Verification items for this drawing (mm, ordinates from the low corner). A direction names the side the tool comes from. Round coordinates to 2 decimals unless told otherwise and drop trailing zeros. Order: outer loops, then holes, each group sorted by start corner. A loop starts at its lowest first (then second) coordinate and runs counter-clockwise, first axis right, second up. Notation, with made-up numbers: (53.25, 67.5) -> (57.25, 67.5) arc R27 cw to (57.25, 97.5) -> close; hole circle Ø4 at (47, 26). An arc over 180 degrees is marked (long way). Answer in a Markdown table with one row per item. Add a question column.
1. Draft check along X on the marked faces 6, 7 and 8. Enter one of: +X half, -X half, draft (parallel to the pull), parting line (faces both ways), or undercut.
2. Sectioned sample at C-C, the plane x = 43.5. Record the boundary of the cut face in (y, z).
3. Sectioned sample at D-D, the plane z = 8. Record the boundary of the cut face in (x, y).
4. Access from +Z, -Z, +X, -X, +Y, -Y to the whole of each face (thin tool, end or side, straight path). Record for the marked faces 1, 2, 3, 4 and 5.
5. Depth check by flat-ended pin: P1, Ø7, axis at x = 28.5, y = 4.5, coming from the +Z side; P2, Ø8, axis at x = 28, y = 23.5, coming from the +Z side; P3, Ø7, axis at x = 22, z = 21.5, coming from the +Y side. Enter the tip coordinate at first touch or a pass-through.
6. Material ranges on L1, parallel to Z at x = 21.5, y = 12.25; L2, parallel to Z at x = 31.5, y = 15.75; L3, parallel to X at y = 2.5, z = 22.25, recorded low to high. Write a range as from..to.
7. Sectioned sample at A-A, the plane y = 23. Record the boundary of the cut face in (x, z).
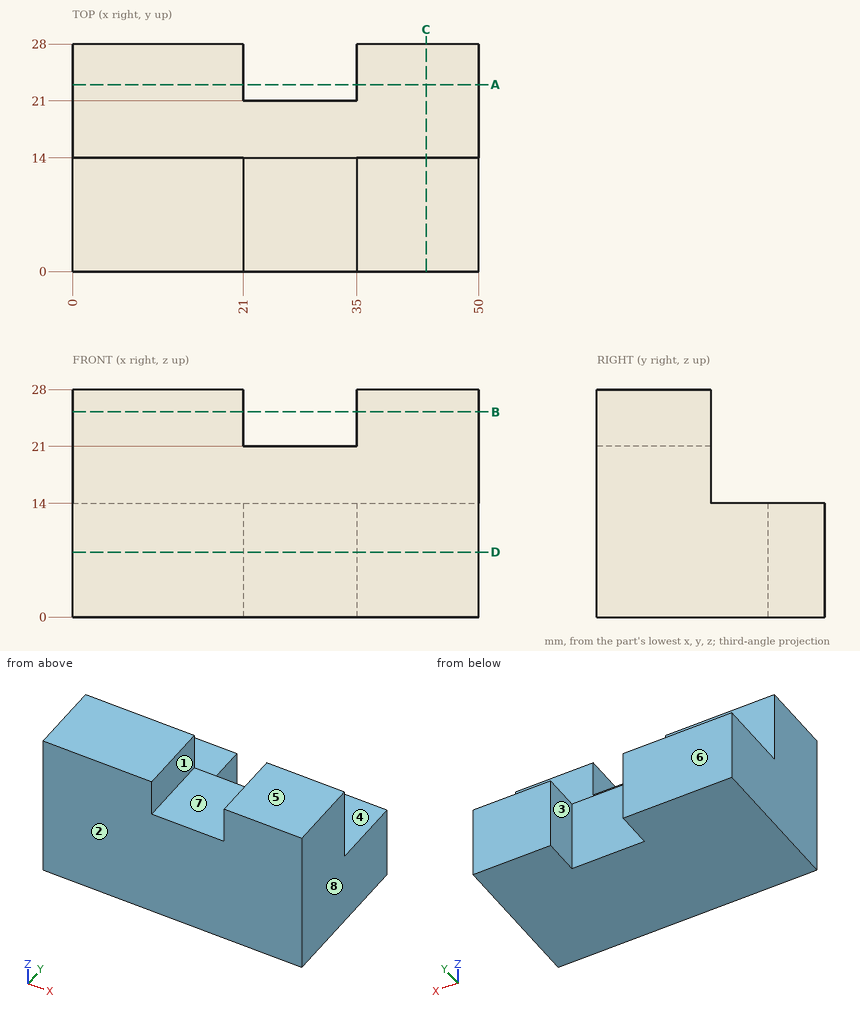
Answer key:
| question | item | result |
|---|---|---|
| 1 | face 6 | draft |
| 1 | face 7 | undercut |
| 1 | face 8 | +X half |
| 2 | outline | (0, 0) -> (28, 0) -> (28, 14) -> (14, 14) -> (14, 28) -> (0, 28) -> close |
| 3 | outline | (0, 0) -> (50, 0) -> (50, 28) -> (35, 28) -> (35, 21) -> (21, 21) -> (21, 28) -> (0, 28) -> close |
| 4 | face 1 | +Z, +Y, -Y |
| 4 | face 2 | +Z, -Z, +X, -X, -Y |
| 4 | face 3 | +Z, -Z, +Y |
| 4 | face 4 | +Z, +X, -X, +Y |
| 4 | face 5 | +Z, +X, -X, +Y, -Y |
| 5 | P1 | stops at z = 21 |
| 5 | P2 | stops at z = 14 |
| 5 | P3 | stops at y = 14 |
| 6 | L1 | z = 0..21 |
| 6 | L2 | z = 0..14 |
| 6 | L3 | x = 0..21, 35..50 |
| 7 | outline | (0, 0) -> (21, 0) -> (21, 14) -> (0, 14) -> close; (35, 0) -> (50, 0) -> (50, 14) -> (35, 14) -> close |
